Here's how the part is built. I have some questions about the finished solid (model axes, mm). Face numbers are marked on the shaded views. A direction names the side the tool comes from. Round coordinates to 2 decimals unless told otherwise and drop trailing zeros. Write each loop counter-clockwise with the first axis right and the second up, starting at its lowest first coordinate (ties: lowest second). Pieces come first, ordered by that corner, then holes. Notation, with made-up numbers: (74.5, 26.25) - (102.5, 26.25) arc R36 cw to (102.5, 62.25) - close; hole circle Ø4 at (63.25, 18.5). An arc over 180 degrees is marked (long way). Write item = value, one per line. Start each with the question number.
Item 1: If I drill on line 1 along X through (y, z) = (16, 1.5); line 2 along Y through (x, z) = (0, 5.15); line 3 along X through (y, z) = (-100, 5.45), over which ranges is the centre line in solid material (lowest first)? Write a range as [from, to].
Item 2: Which directions (+Z, -Z, +X, -X, +Y, -Y) give clear straight access to the entire face, cutting with the end or side of a thin tool? Please do the marked faces 1 and 2.
Item 3: If we section it at B-B (z = 2.25): Give the number of separate pieces and of enclosed holes in the cut face, and give its area (3 significant figures).
Item 4: For P1, Ø4.5, axis at y = -32, z = -2.5, coming from the -X side; P2, Ø3, axis at x = -6, z = -5, coming from the -Y side; P3, Ø1, axis at x = -1.5, y = -33, coming from the -Z side; P4, Ø2, axis at x = 0, y = -100, coming from the -Z side, each with a flat end and sliding along its axis, tell me the tip position at first contact or that it passes through.
Item 5: If we section it at A-A (y = 65): Please give me the cut outline in (x, z).
```python
from build123d import *

# Parameters (mm, degrees)
BOSS_EXTRUDE1_DEPTH                                 = 8
FILLET1_R                                           = 10
CUT_EXTRUDE8_DEPTH                                  = 4
CSK_FOR_M3_COUNTERSUNK_FLAT_HEAD_SCREW2_D           = 3.4
CSK_FOR_M3_COUNTERSUNK_FLAT_HEAD_SCREW2_DEPTH       = 8.5
CSK_FOR_M3_COUNTERSUNK_FLAT_HEAD_SCREW2_CSINK_D     = 6.3
CSK_FOR_M3_COUNTERSUNK_FLAT_HEAD_SCREW2_CSINK_ANGLE = 90
CSK_FOR_M3_COUNTERSUNK_FLAT_HEAD_SCREW2_TIP         = 1.021463052
SKETCH14_W                                          = 9
SKETCH14_H                                          = 24.3
BOSS_EXTRUDE2_DEPTH                                 = 2
FILLET3_R                                           = 1.65
BOSS_EXTRUDE3_REACH                                 = 112.905
SKETCH16_W                                          = 2.15
SKETCH16_H                                          = 5
SKETCH18_W                                          = 2.15
SKETCH18_H                                          = 5
CIRPATTERN1_COUNT                                   = 2
CIRPATTERN2_COUNT                                   = 2
CIRPATTERN2_COPY_1_REACH                            = 112.905
CIRPATTERN2_COPY_1_SKETCH_W                         = 2.15
CIRPATTERN2_COPY_1_SKETCH_H                         = 5
CIRPATTERN2_COPY_2_SKETCH_W                         = 2.15
CIRPATTERN2_COPY_2_SKETCH_H                         = 5
FILLET3_OF_CIRPATTERN2_R                            = 1.65


with BuildPart() as part:
    # Sketch1 → Boss-Extrude1 (new body)
    with BuildSketch(Plane(origin=(0, 0, 0), x_dir=(0, 1, 0), z_dir=(0, 0, 1))):
        with BuildLine():
            Line((100, -10), (-100, -10))
            ThreePointArc((-100, -10), (-110, 0), (-100, 10))
            Line((-100, 10), (100, 10))
            Line((100, 10), (100, -10))
        make_face()
        with BuildLine():
            Line((-6.5, 5.2), (93.5, 5.2))
            ThreePointArc((93.5, 5.2), (95.2, 3.5), (93.5, 1.8))
            Line((93.5, 1.8), (-6.5, 1.8))
            ThreePointArc((-6.5, 1.8), (-8.2, 3.5), (-6.5, 5.2))
        make_face(mode=Mode.SUBTRACT)
        with BuildLine():
            Line((-6.5, -1.8), (93.5, -1.8))
            ThreePointArc((93.5, -1.8), (95.2, -3.5), (93.5, -5.2))
            Line((93.5, -5.2), (-6.5, -5.2))
            ThreePointArc((-6.5, -5.2), (-8.2, -3.5), (-6.5, -1.8))
        make_face(mode=Mode.SUBTRACT)
    extrude(amount=BOSS_EXTRUDE1_DEPTH)

    # Fillet1
    fillet1_edges = [part.edges().sort_by_distance(p)[0] for p in [
        (-10, 100, 4),
        (10, 100, 4),
    ]]
    fillet(fillet1_edges, radius=FILLET1_R - 0.0001)  # a hair under: the kernel refuses the full size

    # Sketch8 → Cut-Extrude8 (cut)
    with BuildSketch(Plane(origin=(0, 0, 0), x_dir=(1, 0, 0), z_dir=(0, 0, -1))):
        with BuildLine():
            Line((-10, 76), (-10, 110))
            Line((-10, 110), (10, 110))
            Line((10, 110), (10, 76))
            ThreePointArc((10, 76), (0, 86), (-10, 76))
        make_face()
    extrude(amount=-CUT_EXTRUDE8_DEPTH, mode=Mode.SUBTRACT)

    # CSK for M3 Countersunk Flat Head Screw2
    with Locations(Plane.XY.offset(8)):
        with Locations((0, -100)):
            CounterSinkHole(CSK_FOR_M3_COUNTERSUNK_FLAT_HEAD_SCREW2_D / 2, CSK_FOR_M3_COUNTERSUNK_FLAT_HEAD_SCREW2_CSINK_D / 2, depth=CSK_FOR_M3_COUNTERSUNK_FLAT_HEAD_SCREW2_DEPTH, counter_sink_angle=CSK_FOR_M3_COUNTERSUNK_FLAT_HEAD_SCREW2_CSINK_ANGLE)
            with Locations((0, 0, -(CSK_FOR_M3_COUNTERSUNK_FLAT_HEAD_SCREW2_DEPTH + CSK_FOR_M3_COUNTERSUNK_FLAT_HEAD_SCREW2_TIP / 2))):  # 118° drill point
                Cone(0, CSK_FOR_M3_COUNTERSUNK_FLAT_HEAD_SCREW2_D / 2, CSK_FOR_M3_COUNTERSUNK_FLAT_HEAD_SCREW2_TIP, mode=Mode.SUBTRACT)

    # Sketch14 → Boss-Extrude2 (add)
    with BuildSketch(Plane.XY):
        with Locations((-5, -22.85)):
            Rectangle(SKETCH14_W, SKETCH14_H)
    boss_extrude2 = extrude(amount=-BOSS_EXTRUDE2_DEPTH)

    # Fillet3
    fillet3_edges = [part.edges().sort_by_distance(p)[0] for p in [
        (-5, -35, -2),
        (-9.5, -22.85, -2),
        (-5, -10.7, -2),
        (-0.5, -22.85, -2),
    ]]
    fillet(fillet3_edges, radius=FILLET3_R)

    # Boss-Extrude3: up to this face of the body (flat: up to its plane)
    boss_extrude3_end = Plane(part.part.faces().sort_by_distance((0.402421267, 0.024510411, 0))[0])
    # Sketch16 → Boss-Extrude3 (add, up to the picked face)
    with BuildSketch(Plane.XY.offset(-2), mode=Mode.PRIVATE) as boss_extrude3_sk1:
        with Locations((-1.575, -32.5)):
            Rectangle(SKETCH16_W, SKETCH16_H)
    boss_extrude3_tool1 = split(extrude(boss_extrude3_sk1.sketch, amount=BOSS_EXTRUDE3_REACH, mode=Mode.PRIVATE), bisect_by=boss_extrude3_end, keep=Keep.BOTH, mode=Mode.PRIVATE)
    boss_extrude3 = boss_extrude3_tool1.solids().sort_by(Axis((-1.575, -32.5, -2), (0, 0, 1)))[0]
    add(boss_extrude3)

    # Sweep3: sweep along a path in Sketch17
    with BuildLine(Plane(origin=(0, -33.35, 0), x_dir=(-1, 0, 0), z_dir=(0, -1, 0))) as sweep3_path:
        Line((2.65, 2), (2.65, 4.35))
        ThreePointArc((2.65, 4.35), (4.405679741, 6.623605821), (7.049390153, 5.5))
    # Sketch18 → Sweep3 (sweep)
    with BuildSketch(Plane.XY.offset(-2)):
        with Locations((-1.575, -32.5)):
            Rectangle(SKETCH18_W, SKETCH18_H)
    sweep3 = sweep(path=sweep3_path.line)

    # CirPattern1: Boss-Extrude3, Sweep3 ×2 about axis
    cirpattern1_axis = Axis((-5, -22.85, 0), (0, 0, 1))
    add([boss_extrude3.rotate(cirpattern1_axis, i * 360 / CIRPATTERN1_COUNT) for i in range(1, CIRPATTERN1_COUNT)])
    add([sweep3.rotate(cirpattern1_axis, i * 360 / CIRPATTERN1_COUNT) for i in range(1, CIRPATTERN1_COUNT)])

    # CirPattern2: Boss-Extrude2, Boss-Extrude3, Sweep3 ×2 about axis
    cirpattern2_axis = Axis((0, -32.5, 0), (0, 0, 1))
    add([boss_extrude2.rotate(cirpattern2_axis, i * 360 / CIRPATTERN2_COUNT) for i in range(1, CIRPATTERN2_COUNT)])
    add([boss_extrude3.rotate(cirpattern2_axis, i * 360 / CIRPATTERN2_COUNT) for i in range(1, CIRPATTERN2_COUNT)])
    add([sweep3.rotate(cirpattern2_axis, i * 360 / CIRPATTERN2_COUNT) for i in range(1, CIRPATTERN2_COUNT)])

    # CirPattern2 copy 1: up to this face of the body (flat: up to its plane)
    cirpattern2_copy_1_end = Plane(part.part.faces().sort_by_distance((10.402421267, -19.275489589, 0))[0])
    # CirPattern2 copy 1 sketch → CirPattern2 copy 1 (add, up to the picked face)
    with BuildSketch(Plane(origin=(10, -19.3, -2), x_dir=(1, 0, 0), z_dir=(0, 0, 1)), mode=Mode.PRIVATE) as cirpattern2_copy_1_sk1:
        with Locations((-1.575, -32.5)):
            Rectangle(CIRPATTERN2_COPY_1_SKETCH_W, CIRPATTERN2_COPY_1_SKETCH_H)
    cirpattern2_copy_1_tool1 = split(extrude(cirpattern2_copy_1_sk1.sketch, amount=CIRPATTERN2_COPY_1_REACH, mode=Mode.PRIVATE), bisect_by=cirpattern2_copy_1_end, keep=Keep.BOTH, mode=Mode.PRIVATE)
    add(cirpattern2_copy_1_tool1.solids().sort_by(Axis((8.425, -51.8, -2), (0, 0, 1)))[0])

    # CirPattern2 copy 2: sweep along a path in CirPattern2 copy 2 path
    with BuildLine(Plane(origin=(10, -52.65, 0), x_dir=(-1, 0, 0), z_dir=(0, -1, 0))) as cirpattern2_copy_2_path:
        Line((2.65, 2), (2.65, 4.35))
        ThreePointArc((2.65, 4.35), (4.405679741, 6.623605821), (7.049390153, 5.5))
    # CirPattern2 copy 2 sketch → CirPattern2 copy 2 (sweep)
    with BuildSketch(Plane(origin=(10, -19.3, -2), x_dir=(1, 0, 0), z_dir=(0, 0, 1))):
        with Locations((-1.575, -32.5)):
            Rectangle(CIRPATTERN2_COPY_2_SKETCH_W, CIRPATTERN2_COPY_2_SKETCH_H)
    sweep(path=cirpattern2_copy_2_path.line)

    # Fillet3 of CirPattern2
    fillet3_of_cirpattern2_edges = [part.edges().sort_by_distance(p)[0] for p in [
        (5, -30, -2),
        (9.5, -42.15, -2),
        (5, -54.3, -2),
        (0.5, -42.15, -2),
    ]]
    fillet(fillet3_of_cirpattern2_edges, radius=FILLET3_OF_CIRPATTERN2_R)


solid = part.part
```
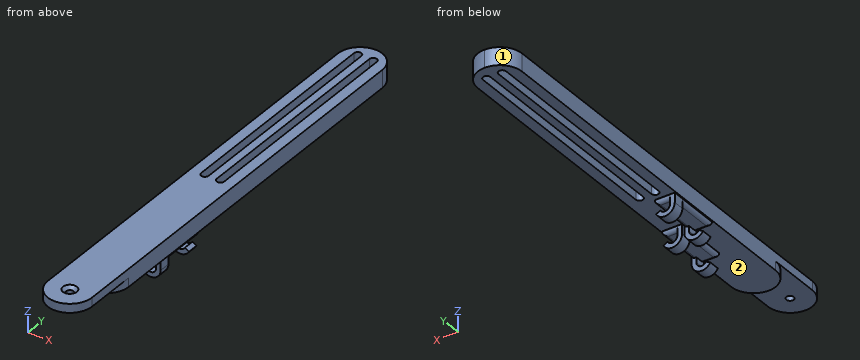
Reply:
q1.line_1 = [-10, -5.2], [-1.8, 1.8], [5.2, 10]
q1.line_2 = [-110, -101.7], [-98.3, 100]
q1.line_3 = [-10, -1.7], [1.7, 10]
q2.face_1 = +Z, -Z, -X, +Y
q2.face_2 = -Z
q3.separate_pieces = 1
q3.enclosed_holes = 2
q3.area = 2,940 mm2
q4.P1 = -9.5
q4.P2 = -35
q4.P3 = -7.7
q4.P4 = through
q5.outline = (-10, 0) - (-5.2, 0) - (-5.2, 8) - (-10, 8) - close; (-1.8, 0) - (1.8, 0) - (1.8, 8) - (-1.8, 8) - close; (5.2, 0) - (10, 0) - (10, 8) - (5.2, 8) - close
